Check sheet for the modelled part. Datum: model origin and axes. Units: mm. Round coordinates to 2 decimals unless told otherwise and drop trailing zeros. Loops run counter-clockwise (first coordinate to the right, second up) from the corner with the lowest first, then second, coordinate; pieces in that order, holes last. Notation, with made-up numbers: M 27,40 L 39,40 A21 ccw 39,57 Z; hole C 36.5,73 d4. An arc over 180 degrees is marked long. Write item = value, one per line. Start each with the question number.
(1) Cross-section at D-D on z = -1.5. Record the boundary of the cut face in (x, y), plus the area to 3 significant figures.
(2) Mould release check, pull along X, two halves, no side actions. Record for faces 1 (the face through (3.31, -10.864, -14.79)), 2 (the face through (-3, -6, 0)), 3 (the face through (-0.75, 5.7, -16.42)): pulls with the +X half, pulls with the -X half, needs draft (parallel to the pull), parting line crosses it, or undercut.
(3) Cross-section at B-B on y = 0. Record the boundary of the cut face in (x, z) (3 decimals), plus the area to 3 significant figures.
(4) Cross-section at A-A on z = -14. Record the boundary of the cut face in (x, y).
(5) Cross-section at C-C on x = 0. Record the boundary of the cut face in (y, z) (3 decimals), plus the area to 3 significant figures.
(6) Scan lines: L1, parallel to Y at x = 0, z = -0.6; L2, parallel to Y at x = 3.5, z = -27; L3, parallel to X at y = 0, z = -12.5. Record each from-to range of solid material in increasing order. Write a range as from..to.
(7) Go/stop test with flat-tipped pins: P1, Ø12, axis at x = 11, z = -12.5, coming from the +Y side; P2, Ø10, axis at x = 11, z = -25, coming from the -Y side; P3, Ø2, axis at x = 1, z = -26, coming from the -Y side; P4, Ø7, axis at x = 0, y = 0, coming from the -Z side. Record where each tip stops, or that it passes through.
from build123d import *

# Parameters (mm, degrees)
F0_R     = 5.75
F1_DEPTH = 30
F2_R     = 2
F5_R     = 0.5


with BuildPart() as f1:
    # F0 (on Top) → F1 (new body)
    with BuildSketch(Plane.XY):
        Polygon((-8.8044720603, 9.3002779725), (-8.8044720603, -15.6997220275), (-5.8044720603, -15.6997220275), (13.2937646807, -5.5672283149), (13.2937646807, 0.4327716851), (1.1955279397, 9.3002779725), align=None)
        Circle(F0_R, mode=Mode.SUBTRACT)
    extrude(amount=-F1_DEPTH)

    # F2
    f2_edges = [f1.edges().sort_by_distance(p)[0] for p in [
        (-8.804472, 9.300278, -15),
        (1.195528, 9.300278, -15),
        (-8.804472, -15.699722, -15),
        (13.293765, -5.567228, -15),
        (-5.804472, -15.699722, -15),
        (13.293765, 0.432772, -15),
    ]]
    fillet(f2_edges, radius=F2_R)

    # F3 (on Right) → F4 (revolve, cut)
    with BuildSketch(Plane.YZ):
        with BuildLine():
            Line((0, 0), (-5.5240949485, 0))
            ThreePointArc((-5.5240949485, 0), (-4.8096582519, -5.3738423941), (0, -7.875))
            Line((0, -7.875), (0, 0))
        make_face()
    revolve(axis=Axis((0, 0, -1), (0, 0, -1)), mode=Mode.SUBTRACT)

    # F5
    f5_edges = [f1.edges().sort_by_distance(p)[0] for p in [
        (-5.75, 0, 0),
    ]]
    fillet(f5_edges, radius=F5_R)


solid = f1.part
Result:
q1.outline = M -8.8,-13.7 A2 ccw -6.8,-15.7 L -6.3,-15.7 A2 ccw -5.36,-15.47 L 12.23,-6.13 A2 ccw 13.29,-4.36 L 13.29,-0.58 A2 ccw 12.48,1.03 L 1.72,8.91 A2 ccw 0.54,9.3 L -6.8,9.3 A2 ccw -8.8,7.3 Z; hole C 0,0 d11.71
q1.area = 292 mm^2
q2.face_1 = pulls with the +X half
q2.face_2 = needs draft
q2.face_3 = undercut
q3.outline = M -8.804,-30 L -5.75,-30 L -5.75,-3.205 A5.875 cw -5.75,-0.795 L -5.75,-0.5 A0.5 ccw -6.25,0 L -8.804,0 Z; M 5.75,-30 L 13.208,-30 L 13.208,0 L 6.25,0 A0.5 ccw 5.75,-0.5 L 5.75,-0.795 A5.875 cw 5.75,-3.205 Z
q3.area = 315 mm^2
q4.outline = M -8.8,-13.7 A2 ccw -6.8,-15.7 L -6.3,-15.7 A2 ccw -5.36,-15.47 L 12.23,-6.13 A2 ccw 13.29,-4.36 L 13.29,-0.58 A2 ccw 12.48,1.03 L 1.72,8.91 A2 ccw 0.54,9.3 L -6.8,9.3 A2 ccw -8.8,7.3 Z; hole C 0,0 d11.5
q5.outline = M -12.62,-30 L -5.75,-30 L -5.75,-3.205 A5.875 cw -5.75,-0.795 L -5.75,-0.5 A0.5 ccw -6.25,0 L -12.62,0 Z; M 5.75,-30 L 9.3,-30 L 9.3,0 L 6.25,0 A0.5 ccw 5.75,-0.5 L 5.75,-0.795 A5.875 cw 5.75,-3.205 Z
q5.area = 312 mm^2
q6.L1 = -12.62..-5.75, 5.75..9.3
q6.L2 = -10.76..-4.56, 4.56..7.61
q6.L3 = -8.8..-5.75, 5.75..13.21
q7.P1 = 6.51
q7.P2 = -9.44
q7.P3 = -12.62
q7.P4 = through
